The listing builds one solid part. Answer for the finished solid, in the listing's coordinates (mm). A direction names the side the tool comes from. Round coordinates to 2 decimals unless told otherwise and drop trailing zeros. Write each loop counter-clockwise with the first axis right and the second up, starting at its lowest first coordinate (ties: lowest second). Pieces come first, ordered by that corner, then holes. Notation, with made-up numbers: M 53,11.25 L 103,11.25 A25 cw 103,50.25 Z; hole C -15,8.25 d2. An arc over 180 degrees is marked long. Write each question's results on one line, items separated by ' | '.
from build123d import *

# Parameters (mm, degrees)
SKETCH_4_W          = 30
SKETCH_4_H          = 3
EXTRUDE_3_DEPTH     = 30
EXTRUDE_START       = -9
SKETCH_5_W          = 20
SKETCH_5_H          = 60
EXTRUDE_4_DEPTH     = 12
SKETCH_6_R          = 7
CUT_EXTRUDE_1_DEPTH = 5
CUT_EXTRUDE_START   = -7
SKETCH_6_5_R        = 7
CUT_EXTRUDE_3_DEPTH = 5
SKETCH_7_R          = 1.5
CUT_EXTRUDE_4_DEPTH = 74.484692283
FILLET_1_R          = 5


with BuildPart() as part:
    # Sketch 4 → Extrude 3 (new body)
    with BuildSketch(Plane.XY):
        with Locations((15, 1.5)):
            Rectangle(SKETCH_4_W, SKETCH_4_H)
    extrude(amount=EXTRUDE_3_DEPTH)

    # Sketch 5 → Extrude 4 (add)
    with BuildSketch(Plane.ZY.offset(EXTRUDE_START)):
        with Locations((15, 33)):
            Rectangle(SKETCH_5_W, SKETCH_5_H)
    extrude(amount=-EXTRUDE_4_DEPTH)

    # Sketch 6 → Cut-Extrude 1 (cut)
    with BuildSketch(Plane.ZY.offset(-9)):
        with Locations((15, 50)):
            Circle(SKETCH_6_R)
    extrude(amount=-CUT_EXTRUDE_1_DEPTH, mode=Mode.SUBTRACT)

    # Sketch 6_5 → Cut-Extrude 3 (cut)
    with BuildSketch(Plane.ZY.offset(-9).offset(CUT_EXTRUDE_START)):
        with Locations((15, 50)):
            Circle(SKETCH_6_5_R)
    extrude(amount=-CUT_EXTRUDE_3_DEPTH, mode=Mode.SUBTRACT)

    # Sketch 7 → Cut-Extrude 4 (cut, through all)
    with BuildSketch(Plane(origin=(0, 3, 0), x_dir=(1, 0, 0), z_dir=(0, 1, 0))):
        with Locations(Location((4, -4, 0), (0, 0, 180))):
            Circle(SKETCH_7_R)
        with Locations(Location((26, -4, 0), (0, 0, 180))):
            Circle(SKETCH_7_R)
        with Locations(Location((26, -26, 0), (0, 0, 180))):
            Circle(SKETCH_7_R)
        with Locations(Location((4, -26, 0), (0, 0, 180))):
            Circle(SKETCH_7_R)
    extrude(amount=-CUT_EXTRUDE_4_DEPTH, mode=Mode.SUBTRACT)

    # Fillet 1
    fillet_1_edges = [part.edges().sort_by_distance(p)[0] for p in [
        (15, 63, 5),
        (15, 63, 25),
    ]]
    fillet(fillet_1_edges, radius=FILLET_1_R)


solid = part.part
1) Section C-C (y = 50) is taken. Determine the outline of the cut face in (x, z), then the cut area to 3 significant figures.
Return value:
outline: M 9,5 L 21,5 L 21,8 L 16,8 L 16,22 L 21,22 L 21,25 L 9,25 L 9,22 L 14,22 L 14,8 L 9,8 Z | area: 100 mm²
2) Section B-B (z = 26) is taken. Determine the outline of the cut face in (x, y).
Return value:
outline: M 0,0 L 2.5,0 L 2.5,3 L 0,3 Z; M 5.5,0 L 24.5,0 L 24.5,3 L 5.5,3 Z; M 27.5,0 L 30,0 L 30,3 L 27.5,3 Z
3) A tool of negligible diameter and unlimited length cuts with its end or side. For faces 5 (the face through (11.46, 54.73, 9.84)), 6 (the face through (18.46, 54.73, 9.84)), 7 (the face through (15, 30, 5)), from which of +Z, -Z, +X, -X, +Y, -Y can it reach the whole face along a straight path? Write none if from no direction.
Return value:
face 5: -X | face 6: +X | face 7: -Z, +X, -X, +Y
4) Each of these flat-tipped pins is pushed along its axis until it touches: pin 1 (11 mm diameter, centred on y = 50, z = 15, fed in from +X); pin 2 (5 mm diameter, centred on y = 23, z = 14.5, fed in from +X); pin 3 (3.5 mm diameter, centred on x = 4, z = 26, fed in from +Y); pin 4 (1.8 mm diameter, centred on x = 4, z = 4, fed in from -Y). Where does it stop, or does it pass through?
Return value:
pin 1: x = 16 | pin 2: x = 21 | pin 3: y = 3 | pin 4: through
5) Find the intervals of material crossed by line 1 (Z direction, x = 26, y = 0.95); line 2 (Y direction, x = 2.5, z = 5.25); line 3 (Y direction, x = 11.85, z = 15), in increasing order.
Return value:
line 1: 0 to 2.5, 5.5 to 24.5, 27.5 to 30 | line 2: 0 to 3 | line 3: 0 to 43, 57 to 63
6) Section A-A (x = 4) is taken. Determine the outline of the cut face in (y, z), then the cut area to 3 significant figures.
Return value:
outline: M 0,0 L 3,0 L 3,2.5 L 0,2.5 Z; M 0,5.5 L 3,5.5 L 3,24.5 L 0,24.5 Z; M 0,27.5 L 3,27.5 L 3,30 L 0,30 Z | area: 72.0 mm²
7) Section D-D (x = 16.75) is taken. Determine the outline of the cut face in (y, z), then the cut area to 3 significant figures.
Return value:
outline: M 0,0 L 3,0 L 3,5 L 58,5 A5 ccw 63,10 L 63,20 A5 ccw 58,25 L 3,25 L 3,30 L 0,30 Z; hole C 50,15 d14 | area: 1,130 mm²
8) The mould has two halves that part along X. Classify faces 1 (the face through (30, 1, 15)), 2 (the face through (0, 1, 15)), 3 (the face through (15, 61, 6)), 4 (the face through (2.57, 1.52, 4.45)): +X half, -X half, draft (parallel to the pull), parting line (faces both ways), or undercut.
Return value:
face 1: +X half | face 2: -X half | face 3: draft | face 4: undercut
